Source: CAD feature listing. Evaluate the final solid. Frame: model axes, mm. Face numbers are marked on the shaded views. Round coordinates to 2 decimals unless told otherwise and drop trailing zeros. Write each loop counter-clockwise with the first axis right and the second up, starting at its lowest first coordinate (ties: lowest second). Pieces come first, ordered by that corner, then holes.
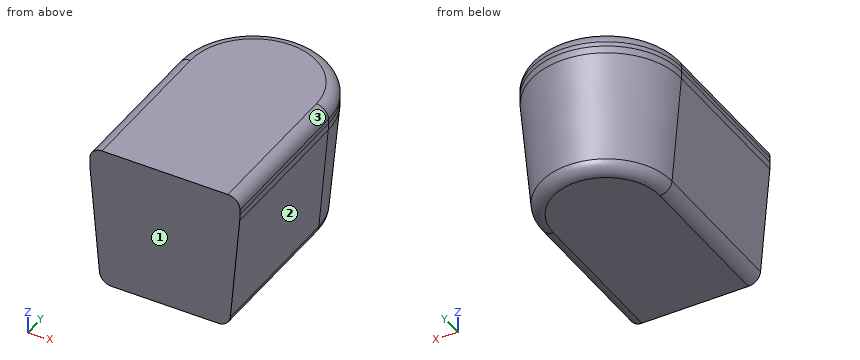
from build123d import *

# Parameters (mm, degrees)
F1_DEPTH    = 350
F2_SIZE2    = 26.2465990578
F2_SIZE     = 300
F3_T1_DEPTH = 396.8304714543
F3_T4_ANGLE = 180
F4_R        = 30


# Not quite as in the source:
# - a fillet or chamfer that OpenCascade refuses, or shapes differently, is made with other operations: its cross-section is extruded or revolved along the edge and cut away or added


with BuildPart() as f1:
    # F0 (on Top) → F1 (new body)
    with BuildSketch(Plane.XY):
        with BuildLine():
            Line((-185, 375), (-185, 0))
            Line((-185, 0), (185, 0))
            Line((185, 0), (185, 375))
            ThreePointArc((185, 375), (130.8147545195, 505.8147545195), (0, 560))
            ThreePointArc((0, 560), (-130.8147545195, 505.8147545195), (-185, 375))
        make_face()
    extrude(amount=F1_DEPTH)

    # F2
    f2_edges = [f1.edges().sort_by_distance(p)[0] for p in [
        (185, 187.5, 0),
        (0, 560, 0),
        (-185, 187.5, 0),
    ]]
    chamfer(f2_edges, length=F2_SIZE, length2=F2_SIZE2)

    # F3: fillet of radius 200 on 3 edges, made by hand

    # F3_s2 → F3_t1 (cut)
    with BuildSketch(Plane.XZ.offset(-375)):
        with BuildLine():
            ThreePointArc((-185, 308.7321885817), (-184.8096443164, 300.0083111086), (-184.2389396183, 291.3010400322))
            Line((-184.2389396183, 291.3010400322), (-185, 300))
            Line((-185, 300), (-185, 308.7321885817))
        make_face()
        with BuildLine():
            ThreePointArc((185, 308.7321885817), (184.8096443164, 300.0083111086), (184.2389396183, 291.3010400322))
            Line((184.2389396183, 291.3010400322), (185, 300))
            Line((185, 300), (185, 308.7321885817))
        make_face()
    extrude(amount=F3_T1_DEPTH, mode=Mode.SUBTRACT)

    # F3_s3 → F3_t4 (revolve, cut)
    with BuildSketch(Plane.XZ.offset(-375)):
        with BuildLine():
            ThreePointArc((185, 308.7321885817), (184.8096443164, 300.0083111086), (184.2389396183, 291.3010400322))
            Line((184.2389396183, 291.3010400322), (185, 300))
            Line((185, 300), (185, 308.7321885817))
        make_face()
    revolve(axis=Axis((0, 375, 300), (0, 0, 1)), revolution_arc=F3_T4_ANGLE, mode=Mode.SUBTRACT)

    # F4
    f4_edges = [f1.edges().sort_by_distance(p)[0] for p in [
        (158.753401, 187.5, 0),
        (0, 533.753401, 0),
        (-158.753401, 187.5, 0),
        (185, 187.5, 350),
        (0, 560, 350),
        (-185, 187.5, 350),
    ]]
    fillet(f4_edges, radius=F4_R)


solid = f1.part
1) Section query A-A on y = 199. Return the cut outline in (x, z).
Taken from the geometry:
outline: (-185, 308.73) arc R200 ccw to (-184.24, 291.3) - (-161.15, 27.39) arc R30 ccw to (-131.26, 0) - (131.26, 0) arc R30 ccw to (161.15, 27.39) - (184.24, 291.3) arc R200 ccw to (185, 308.73) - (185, 320) arc R30 ccw to (155, 350) - (-155, 350) arc R30 ccw to (-185, 320) - close
2) Section query C-C on z = 174.5. Return the cut outline in (x, y), then the cut area to 3 significant figures.
Taken from the geometry:
outline: (-174.02, 0) - (174.02, 0) - (174.02, 375) arc R174.02 ccw to (-174.02, 375) - close
area: 178,000 mm2
3) Section query B-B on z = 243.5. Return the cut outline in (x, y).
Taken from the geometry:
outline: (-180.06, 0) - (180.06, 0) - (180.06, 375) arc R180.06 ccw to (-180.06, 375) - close
4) Contact query for flat-ended pins moving along their axis: P1, Ø2, axis at x = 35, z = 190, coming from the +Y side; P2, Ø12, axis at y = 317, z = 90, coming from the -X side; P3, Ø6, axis at x = -126.5, z = 261.5, coming from the +Y side. Output: stop coordinate, or through.
Taken from the geometry:
P1: stops at y = 547.07
P2: stops at x = -167.15
P3: stops at y = 508.21
5) Material intervals for line 1 (X direction, y = 386.5, z = 324.5); line 2 (X direction, y = 471.5, z = 103); line 3 (Y direction, x = -140.5, z = 85.5), sorted ascending.
Taken from the geometry:
line 1: x = -184.3 to 184.3
line 2: x = -137.23 to 137.23
line 3: y = 0 to 463.84
6) Pull-direction query (Z, two-part tool) for the marked faces 1, 2 and 3; classes: released by +Z, released by -Z, zero draft, split by the parting line, or undercut.
Taken from the geometry:
face 1: zero draft
face 2: released by -Z
face 3: released by +Z
